Source: three-view drawing plus pictorial views. Frame: mm from the lowest corner of the part. A direction names the side the tool comes from. Round coordinates to 2 decimals unless told otherwise and drop trailing zeros. Order: outer loops, then holes, each group sorted by start corner. A loop starts at its lowest first (then second) coordinate and runs counter-clockwise, first axis right, second up. Notation, with made-up numbers: (67, 76) - (90, 76) arc R18 ccw to (90, 109) - close; hole circle Ø5 at (46.5, 56.25). An arc over 180 degrees is marked (long way). Use one line per item in the form item = value. Start each with the question number.
Q1. Set-up query: the marked faces 4, 5 and 6. Return all of +Z, -Z, +X, -X, +Y, -Y with unobstructed straight access to the full face (end or side cutting, diameter ignored); none if empty.
Q2. Ray query, line 1 (Y direction, x = 26, z = 28.5) (1 decimal); line 2 (Z direction, x = 3, y = 13.5) (1 decimal); line 3 (Y direction, x = 28, z = 5) (1 decimal). Return the intervals inside material, ascending. Write a range as [from, to].
Q3. Cut plane A-A, the plane x = 12.5. Return the cut outline in (y, z) (1 decimal).
Q4. Cut plane B-B, the plane y = 24. Return the cut outline in (x, z) (1 decimal).
Q5. Cut plane D-D, the plane x = 25. Return the cut outline in (y, z) (1 decimal).
Q6. Pin query (flat end, axial travel): pin 1 Ø3 at (y, z) = (35.5, 15.5) entering from -X (1 decimal); pin 2 Ø5 at (x, y) = (25, 6.5) entering from -Z; pin 3 Ø2 at (x, z) = (28, 15) entering from +Y; pin 4 Ø3 at (x, y) = (11, 18) entering from -Z. Return the tip coordinate at first contact, or that it passes through.
Q7. Draft query along Y for the marked faces 1, 2 and 3. Return one class per face: released by +Y, released by -Y, zero draft, split by the parting line, or undercut.
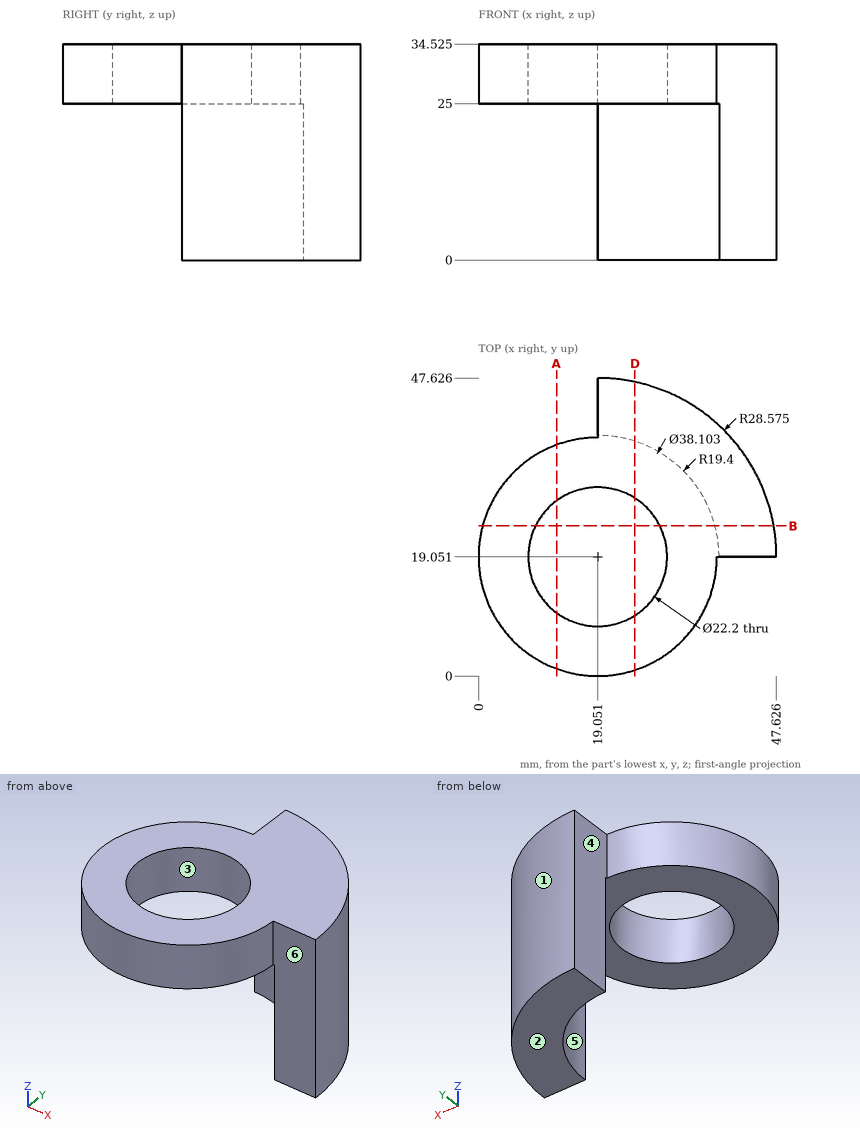
Completed:
q1.face_4 = +Z, -Z, -X, +Y
q1.face_5 = -Z, -X, -Y
q1.face_6 = +Z, -Z, +X, -Y
q2.line_1 = [1.3, 10.4], [27.7, 46.8]
q2.line_2 = [25, 34.5]
q2.line_3 = [36.3, 46.2]
q3.outline = (1.2, 25) - (10.1, 25) - (10.1, 34.5) - (1.2, 34.5) - close; (28, 25) - (36.9, 25) - (36.9, 34.5) - (28, 34.5) - close
q4.outline = (0.7, 25) - (9.1, 25) - (9.1, 34.5) - (0.7, 34.5) - close; (29, 25) - (37.8, 25) - (37.8, 0) - (47.2, 0) - (47.2, 34.5) - (29, 34.5) - close
q5.outline = (1, 25) - (9.7, 25) - (9.7, 34.5) - (1, 34.5) - close; (28.4, 25) - (37.5, 25) - (37.5, 0) - (47, 0) - (47, 34.5) - (28.4, 34.5) - close
q6.pin_1 = 26.4
q6.pin_2 = 25
q6.pin_3 = 46.5
q6.pin_4 = through
q7.face_1 = released by +Y
q7.face_2 = zero draft
q7.face_3 = undercut
